```python
from build123d import *

# Parameters (mm, degrees)
F0_W      = 25.4
F0_H      = 127
F1_DEPTH  = 25.4
F2_W      = 50.8
F2_H      = 25.4
F3_DEPTH  = 25.4
F4_R      = 5.08
F5_DEPTH  = 25.4
F6_R      = 11.0109
F7_DEPTH  = 5.08
F8_R      = 11.0109
F9_DEPTH  = 5.08
F10_DEPTH = 25.4
F11_W     = 25.4
F11_H     = 127
F12_DEPTH = 12.7
F13_DEPTH = 12.7
F14_R     = 13.83665
F15_DEPTH = 25.4
F17_DEPTH = 5.08


with BuildPart() as f1:
    # F0 (on Front) → F1 (new body)
    with BuildSketch(Plane.XZ):
        with Locations((-12.3247115396, -29.6700978652)):
            Rectangle(F0_W, F0_H)
    extrude(amount=F1_DEPTH)

    # F2 (on face) → F3 (join)
    with BuildSketch(Plane.XY.offset(33.8299021348)):
        with Locations((-12.3247115396, -12.7)):
            Rectangle(F2_W, F2_H)
    extrude(amount=F3_DEPTH)

    # F4 (on face) → F5 (cut)
    with BuildSketch(Plane.XZ.offset(25.4)):
        with Locations((-12.3247115396, 46.5299021348)):
            Circle(F4_R)
    extrude(amount=-F5_DEPTH, mode=Mode.SUBTRACT)

    # F6 (on face) → F7 (cut)
    with BuildSketch(Plane.XZ.offset(25.4)):
        with Locations((-12.3247115396, 46.5299021348)):
            Circle(F6_R)
    extrude(amount=-F7_DEPTH, mode=Mode.SUBTRACT)

    # F8 (on face) → F9 (cut)
    with BuildSketch(Plane(origin=(0, 0, 0), x_dir=(-1, 0, 0), z_dir=(0, 1, 0))):
        with Locations((12.3247115396, 46.5299021348)):
            Circle(F8_R)
    extrude(amount=-F9_DEPTH, mode=Mode.SUBTRACT)

    # F4 (on face) → F10 (cut)
    with BuildSketch(Plane.XZ.offset(25.4)):
        with Locations((-12.3247115396, 46.5299021348)):
            Circle(F4_R)
    extrude(amount=-F10_DEPTH, mode=Mode.SUBTRACT)

    # F11 (on face) → F12 (join)
    with BuildSketch(Plane(origin=(-25.0247115396, 0, 0), x_dir=(0, -1, 0), z_dir=(-1, 0, 0))):
        with Locations((12.7, -29.6700978652)):
            Rectangle(F11_W, F11_H)
    extrude(amount=F12_DEPTH)

    # F13 (add): a face of the model
    f13_faces = [f1.faces().sort_by_distance(p)[0] for p in [
        (0.3752884604, -12.7, -29.6700978652),
    ]]
    extrude(f13_faces, amount=F13_DEPTH)

    # F14 (on face) → F15 (cut)
    with BuildSketch(Plane.XZ.offset(25.4)):
        with Locations((-12.3247115396, -67.7700978652)):
            Circle(F14_R)
    extrude(amount=-F15_DEPTH, mode=Mode.SUBTRACT)

    # F16 (on face) → F17 (join)
    with BuildSketch(Plane(origin=(0, 0, -93.1700978652), x_dir=(1, 0, 0), z_dir=(0, 0, -1))):
        with BuildLine():
            ThreePointArc((-37.7247115396, -6.35), (-35.8648396001, -1.8598719395), (-31.3747115396, 0))
            Line((-31.3747115396, 0), (6.7252884604, 0))
            ThreePointArc((6.7252884604, 0), (11.2154165209, -1.8598719395), (13.0752884604, -6.35))
            Line((13.0752884604, -6.35), (13.0752884604, -50.8))
            Line((13.0752884604, -50.8), (38.4752884604, -50.8))
            Line((38.4752884604, -50.8), (38.4752884604, 0))
            Line((38.4752884604, 0), (38.4752884604, 25.4))
            Line((38.4752884604, 25.4), (38.4752884604, 76.2))
            Line((38.4752884604, 76.2), (13.0752884604, 76.2))
            Line((13.0752884604, 76.2), (13.0752884604, 31.75))
            ThreePointArc((13.0752884604, 31.75), (11.2154165209, 27.2598719395), (6.7252884604, 25.4))
            Line((6.7252884604, 25.4), (-31.3747115396, 25.4))
            ThreePointArc((-31.3747115396, 25.4), (-35.8648396001, 27.2598719395), (-37.7247115396, 31.75))
            Line((-37.7247115396, 31.75), (-37.7247115396, 76.2))
            Line((-37.7247115396, 76.2), (-63.1247115396, 76.2))
            Line((-63.1247115396, 76.2), (-63.1247115396, 25.4))
            Line((-63.1247115396, 25.4), (-63.1247115396, 0))
            Line((-63.1247115396, 0), (-63.1247115396, -50.8))
            Line((-63.1247115396, -50.8), (-37.7247115396, -50.8))
            Line((-37.7247115396, -50.8), (-37.7247115396, -6.35))
        make_face()
    extrude(amount=F17_DEPTH)


solid = f1.part
```
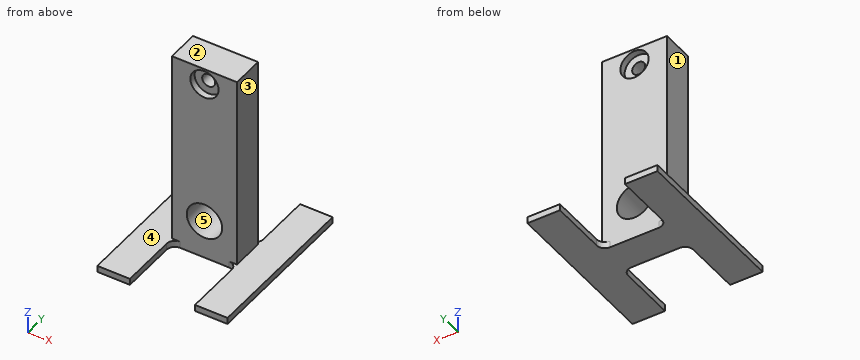
Work out the finished part from the listing and answer in its coordinate system (mm). Face numbers are marked on the shaded views. A direction names the side the tool comes from. Give positions to 0.01 mm unless a question says otherwise; leave off trailing zeros. Order: outer loops, then holes, each group sorted by start corner. A loop starts at its lowest first (then second) coordinate and runs counter-clockwise, first axis right, second up. Notation, with made-up numbers: (13, 63.25) - (59, 63.25) arc R23 cw to (59, 96.25) - close; hole circle Ø2 at (-15, 56.25). An arc over 180 degrees is marked (long way). One line per item, written item: value. Start each with the question number.
1. For a pull along X with two mould halves and no side action, classify the marked faces 3, 4 and 5 as released by +X, released by -X, zero draft, split by the parting line, or undercut.
2. Section A-A, the plane y = -61.5 is taken. Write down the section's boundary in (x, z), then the cut area to 3 significant figures.
3. Each of these flat-tipped pins is pushed along its axis until it touches: pin 1 Ø11 at (x, z) = (-16, 46) entering from +Y; pin 2 Ø6.5 at (x, z) = (-11.5, 42.5) entering from -Y; pin 3 Ø12 at (x, z) = (-27.5, -67.5) entering from +Y. Where does it stop, or does it pass through?
4. Section B-B, the plane x = -20 is taken. Write down the section's boundary in (y, z), then the cut area to 3 significant figures.
5. Consider line 1 (Y direction, x = -8, z = -91); line 2 (X direction, y = -24.5, z = -20.5); line 3 (Z direction, x = 33, y = -33). Determine where each line is inside the solid, lowest interval first.
6. Section D-D, the plane z = 11 is taken. Write down the section's boundary in (x, y).
7. Section C-C, the plane y = -14.5 is taken. Write down the section's boundary in (x, z).
8. Which of the six approach directions +Z, -Z, +X, -X, +Y, -Y give full straight-line access (tool end or side, diameter ignored) to the marked faces 1 and 2?
Filled sheet:
1. face 3: released by +X
1. face 4: zero draft
1. face 5: undercut
2. outline: (-63.12, -98.25) - (-37.72, -98.25) - (-37.72, -93.17) - (-63.12, -93.17) - close; (13.08, -98.25) - (38.48, -98.25) - (38.48, -93.17) - (13.08, -93.17) - close
2. area: 258 mm²
3. pin 1: y = -5.08
3. pin 2: y = -20.32
3. pin 3: y = 0
4. outline: (-25.4, -98.25) - (0, -98.25) - (0, -79.28) - (-25.4, -79.28) - close; (-25.4, -56.26) - (0, -56.26) - (0, 38.63) - (-5.08, 38.63) - (-5.08, 54.42) - (0, 54.42) - (0, 59.23) - (-25.4, 59.23) - (-25.4, 54.42) - (-20.32, 54.42) - (-20.32, 38.63) - (-25.4, 38.63) - close
4. area: 3,250 mm²
5. line 1: -25.4 to 0
5. line 2: -37.72 to 13.08
5. line 3: -98.25 to -93.17
6. outline: (-37.72, -25.4) - (13.08, -25.4) - (13.08, 0) - (-37.72, 0) - close
7. outline: (-63.12, -98.25) - (38.48, -98.25) - (38.48, -93.17) - (13.08, -93.17) - (13.08, 59.23) - (-37.72, 59.23) - (-37.72, -93.17) - (-63.12, -93.17) - close; hole circle Ø27.67 at (-12.32, -67.77); hole circle Ø10.16 at (-12.32, 46.53)
8. face 1: +Z, -X, +Y, -Y
8. face 2: +Z, +X, -X, +Y, -Y
